Part model, mm, in its own coordinate system. A direction names the side the tool comes from. Round coordinates to 2 decimals unless told otherwise and drop trailing zeros. Loops run counter-clockwise (first coordinate to the right, second up) from the corner with the lowest first, then second, coordinate; pieces in that order, holes last. Notation, with made-up numbers: (11, 87.5) - (15, 87.5) arc R24 ccw to (15, 107.5) - close; hole circle Ø2 at (-6.5, 47). An arc over 180 degrees is marked (long way). Write each question's results on one line, items separated by ' | '. Start each with the question number.
(1) Drill centre lines: L1, parallel to Y at x = -127, z = 0; L2, parallel to X at y = 231, z = -36.5; L3, parallel to Y at x = 14, z = -81. Where is each one in solid material? Low to high.
(2) Tool access for faces 4 (the face through (-160, 198, 17)), 5 (the face through (2, 0, -2)), 6 (the face through (-100, 187, 2)), 7 (the face through (166, 160, 1)): list every direction of +Z, -Z, +X, -X, +Y, -Y with a clear straight run to the whole face (end or side of a thin tool).
(3) Mould opens along Z. For faces 1 (the face through (-130, 260, -2)), 2 (the face through (130.42, 229.83, 2.6)), 3 (the face through (-174.83, 102.93, -7.69)) say: released by +Z, released by -Z, zero draft, split by the parting line, or undercut.
(4) Flat gauge pins, fed straight in: P1, Ø3, axis at y = 151, z = 65, coming from the -X side; P2, Ø1, axis at x = -81, y = 73.5, coming from the -Z side; P3, Ø12, axis at x = -137, y = 70.5, coming from the +Z side; P4, Ø1.5, axis at x = 32, z = -43.5, coming from the -Y side. Where does each tip first touch, or does it go through?
(5) Cut at B-B, the plane z = 0. List the corners of the cut face in (x, y).
(6) Cut at D-D, the plane x = -132. List the corners of the cut face in (y, z), then the cut area to 3 significant figures.
(7) Cut at C-C, the plane y = 237. List the corners of the cut face in (x, z).
(8) Cut at A-A, the plane y = 210. List the corners of the cut face in (x, z), then the cut area to 3 significant figures.
from build123d import *

# Parameters (mm, degrees)
ESBO_O1_W                  = 175
ESBO_O1_H                  = 260
ESBO_O2_W                  = 200
ESBO_O2_H                  = 100
ESBO_O2_W_2                = 15
CORTE_EXTRUS_O1_DEPTH      = 176
CORTE_EXTRUS_O1_DEPTH_BACK = 176
ESBO_O3_R                  = 20
CORTE_EXTRUS_O2_DEPTH      = 16
CORTE_EXTRUS_O2_DEPTH_BACK = 336


with BuildPart() as part:
    # Esboço1 → Revolução1 (revolve)
    with BuildSketch(Plane.XY):
        with Locations((87.5, 130)):
            Rectangle(ESBO_O1_W, ESBO_O1_H)
    revolve(axis=Axis((0, 0, 0), (0, 1, 0)))

    # Esboço2 → Corte-extrusão1 (cut, two sides)
    with BuildSketch(Plane.XY) as corte_extrus_o1_sk:
        with Locations((0, 210)):
            Rectangle(ESBO_O2_W, ESBO_O2_H)
        with Locations((167.5, 210)):
            Rectangle(ESBO_O2_W_2, ESBO_O2_H)
        with Locations((-167.5, 210)):
            Rectangle(ESBO_O2_W_2, ESBO_O2_H)
    extrude(amount=CORTE_EXTRUS_O1_DEPTH, mode=Mode.SUBTRACT)
    extrude(corte_extrus_o1_sk.sketch, amount=-CORTE_EXTRUS_O1_DEPTH_BACK, mode=Mode.SUBTRACT)

    # Esboço3 → Corte-extrusão2 (cut, two sides)
    with BuildSketch(Plane(origin=(160, 0, 0), x_dir=(0, 0, -1), z_dir=(1, 0, 0))) as corte_extrus_o2_sk:
        with Locations((0, 210)):
            Circle(ESBO_O3_R)
    extrude(amount=CORTE_EXTRUS_O2_DEPTH, mode=Mode.SUBTRACT)
    extrude(corte_extrus_o2_sk.sketch, amount=-CORTE_EXTRUS_O2_DEPTH_BACK, mode=Mode.SUBTRACT)


solid = part.part
A:
1) L1: 0 to 190, 230 to 260 | L2: -160 to -100, 100 to 160 | L3: 0 to 160
2) face 4: +Z, -Z, -X, +Y | face 5: +Z, -Z, +X, -X, -Y | face 6: +Z, -Z, +Y | face 7: +Z, -Z, +X, +Y
3) face 1: zero draft | face 2: undercut | face 3: split by the parting line
4) P1: x = -163.07 | P2: z = -155.39 | P3: z = 116.03 | P4: y = 0
5) outline: (-175, 0) - (175, 0) - (175, 160) - (160, 160) - (160, 190) - (100, 190) - (100, 160) - (-100, 160) - (-100, 190) - (-160, 190) - (-160, 160) - (-175, 160) - close; (-160, 230) - (-100, 230) - (-100, 260) - (-160, 260) - close; (100, 230) - (160, 230) - (160, 260) - (100, 260) - close
6) outline: (0, -114.9) - (260, -114.9) - (260, 114.9) - (0, 114.9) - close; hole circle Ø40 at (210, 0) | area: 58,500 mm2
7) outline: (-160, -70.89) arc R175 ccw to (-100, -143.61) - (-100, 143.61) arc R175 ccw to (-160, 70.89) - close; (100, -143.61) arc R175 ccw to (160, -70.89) - (160, 70.89) arc R175 ccw to (100, 143.61) - close
8) outline: (-160, -70.89) arc R175 ccw to (-100, -143.61) - (-100, -20) - (-160, -20) - close; (-160, 20) - (-100, 20) - (-100, 143.61) arc R175 ccw to (-160, 70.89) - close; (100, -143.61) arc R175 ccw to (160, -70.89) - (160, -20) - (100, -20) - close; (100, 20) - (160, 20) - (160, 70.89) arc R175 ccw to (100, 143.61) - close | area: 22,600 mm2
